```python
from build123d import *

# Parameters (mm, degrees)
F17_DEPTH = 1
F18_DEPTH = 1
F19_DEPTH = 1
F20_DEPTH = 1
F21_DEPTH = 1
F22_DEPTH = 1
F23_DEPTH = 1
F24_DEPTH = 1


with BuildPart() as f17:
    # F4 (on face) → F17 (new body)
    with BuildSketch(Plane(origin=(0, -27.6923076923, 18.4615384615), x_dir=(-1, 0, 0), z_dir=(0, 0.8320502943, -0.5547001962))):
        Polygon((0, -5.0769823397), (0, 49.9230176603), (-5.5, 49.9230176603), (-7, -5.0769823397), align=None)
    extrude(amount=-F17_DEPTH)



with BuildPart() as f18:
    # F6 (on face) → F18 (new body)
    with BuildSketch(Plane(origin=(20.2323563967, -11.4858345379, 8.3203939199), x_dir=(0.4299219493, 0.8853858987, 0.1768019455), z_dir=(0.8188475708, -0.4648567634, 0.3367444808))):
        Polygon((12.9726874522, 53.3990429211), (-21.4851809627, 10.5049255587), (8.4396185165, 12.6277482381), (24.455774925, 43.748203471), align=None)
    extrude(amount=F18_DEPTH)


with BuildPart() as f19:
    # F8 (on face) → F19 (new body)
    with BuildSketch(Plane(origin=(4.8053501819, -15.3618907739, 7.6432203914), x_dir=(-0.9629489756, -0.2414490977, 0.1201316097), z_dir=(-0.2696836488, 0.8621329558, -0.4289492931))):
        Polygon((-14.8009827937, 17.4534178176), (-9.6599579922, 52.0737855798), (-18.5647011331, 53.379752499), (-28.2916584396, 46.352213701), (-42.6343822268, 48.4820668331), (-46.8858296731, 57.5333205922), (-67.1688557163, 60.5080230193), (-62.6933705008, 27.8129158611), align=None)
    extrude(amount=-F19_DEPTH)


with BuildPart() as f20:
    # F10 (on 3pt) → F20 (new body)
    with BuildSketch(Plane(origin=(-9.1548198434, 27.6665002624, 29.3655492724), x_dir=(0.9752092929, 0.1517429862, 0.161061793), z_dir=(-0.2212845115, 0.6687371352, 0.7098054726))):
        Polygon((32.6463562181, -27.0957188494), (23.8535633809, -29.0158214828), (15.0273586911, -41.144222481), (27.5314988539, -50.3037245848), (69.2506974563, -42.194565074), (80.6394600631, -16.615353079), (60.611431934, -20.9889201884), (54.5101233323, -27.6051149669), (43.7738027725, -29.9991535705), align=None)
    extrude(amount=-F20_DEPTH)


with BuildPart() as f21:
    # F12 (on 3pt) → F21 (new body)
    with BuildSketch(Plane(origin=(0, 25.9269177768, 14.9071230511), x_dir=(-1, 0, 0), z_dir=(0, 0.866918652, 0.4984496473))):
        Polygon((-5.5, 52.0151191187), (0, 52.0151191187), (0, 61.5834322338), (-17.6941536866, 61.5834322338), align=None)
    extrude(amount=-F21_DEPTH)


with BuildPart() as f22:
    # F14 (on face) → F22 (new body)
    with BuildSketch(Plane(origin=(0, -4.8915048648, 0.0087522318), x_dir=(1, 0, 0), z_dir=(0, -0.9999983993, 0.001789269))):
        Polygon((0, 85.6087991728), (0, 68.2863061845), (17.6941536866, 68.2863061845), (25.5, 85.6087991728), align=None)
    extrude(amount=F22_DEPTH)


with BuildPart() as f23:
    # F16 (on 3pt) → F23 (new body)
    with BuildSketch(Plane(origin=(0.2488682272, -0.8172223653, -0.1106827247), x_dir=(-0.9573575318, -0.2862919438, -0.0387747249), z_dir=(-0.2889057916, 0.9486959304, 0.1284892032))):
        Polygon((-60.7194634198, 67.8234958605), (-18.2223306139, 68.3171589865), (-26.3758637032, 85.4787410279), (-69.3695216955, 84.7402476712), align=None)
    extrude(amount=-F23_DEPTH)


with BuildPart() as f17_1:
    add(f17.part)

    add(f18.part)  # F24 merges F18

    add(f19.part)  # F24 merges F19

    add(f20.part)  # F24 merges F20

    add(f21.part)  # F24 merges F21

    add(f22.part)  # F24 merges F22

    add(f23.part)  # F24 merges F23
    # F4 (on face) + F6 (on face) + F8 (on face) + F10 (on 3pt) + F12 (on 3pt) + F14 (on face) + F16 (on 3pt) → F24 (join)
    with BuildSketch(Plane(origin=(0, -27.6923076923, 18.4615384615), x_dir=(-1, 0, 0), z_dir=(0, 0.8320502943, -0.5547001962))):
        Polygon((0, -5.0769823397), (0, 49.9230176603), (-5.5, 49.9230176603), (-7, -5.0769823397), align=None)
    with BuildSketch(Plane(origin=(20.2323563967, -11.4858345379, 8.3203939199), x_dir=(0.4299219493, 0.8853858987, 0.1768019455), z_dir=(0.8188475708, -0.4648567634, 0.3367444808))):
        Polygon((12.9726874522, 53.3990429211), (-21.4851809627, 10.5049255587), (8.4396185165, 12.6277482381), (24.455774925, 43.748203471), align=None)
    with BuildSketch(Plane(origin=(4.8053501819, -15.3618907739, 7.6432203914), x_dir=(-0.9629489756, -0.2414490977, 0.1201316097), z_dir=(-0.2696836488, 0.8621329558, -0.4289492931))):
        Polygon((-14.8009827937, 17.4534178176), (-9.6599579922, 52.0737855798), (-18.5647011331, 53.379752499), (-28.2916584396, 46.352213701), (-42.6343822268, 48.4820668331), (-46.8858296731, 57.5333205922), (-67.1688557163, 60.5080230193), (-62.6933705008, 27.8129158611), align=None)
    with BuildSketch(Plane(origin=(-9.1548198434, 27.6665002624, 29.3655492724), x_dir=(0.9752092929, 0.1517429862, 0.161061793), z_dir=(-0.2212845115, 0.6687371352, 0.7098054726))):
        Polygon((32.6463562181, -27.0957188494), (23.8535633809, -29.0158214828), (15.0273586911, -41.144222481), (27.5314988539, -50.3037245848), (69.2506974563, -42.194565074), (80.6394600631, -16.615353079), (60.611431934, -20.9889201884), (54.5101233323, -27.6051149669), (43.7738027725, -29.9991535705), align=None)
    with BuildSketch(Plane(origin=(0, 25.9269177768, 14.9071230511), x_dir=(-1, 0, 0), z_dir=(0, 0.866918652, 0.4984496473))):
        Polygon((-5.5, 52.0151191187), (0, 52.0151191187), (0, 61.5834322338), (-17.6941536866, 61.5834322338), align=None)
    with BuildSketch(Plane(origin=(0, -4.8915048648, 0.0087522318), x_dir=(1, 0, 0), z_dir=(0, -0.9999983993, 0.001789269))):
        Polygon((0, 85.6087991728), (0, 68.2863061845), (17.6941536866, 68.2863061845), (25.5, 85.6087991728), align=None)
    with BuildSketch(Plane(origin=(0.2488682272, -0.8172223653, -0.1106827247), x_dir=(-0.9573575318, -0.2862919438, -0.0387747249), z_dir=(-0.2889057916, 0.9486959304, 0.1284892032))):
        Polygon((-60.7194634198, 67.8234958605), (-18.2223306139, 68.3171589865), (-26.3758637032, 85.4787410279), (-69.3695216955, 84.7402476712), align=None)
    extrude(amount=-F24_DEPTH, dir=(0, 0.8320502943, -0.5547001962))

    # F25: F17 across plane


with BuildPart() as f17_2:
    add(f17_1.part)
    add(f17_1.part.mirror(Plane.YZ))


solid = f17_2.part
```
For this review, take the finished solid that the model builds, in its own axes (mm). A direction names the side the tool comes from. Give positions to 0.01 mm unless a question says otherwise; leave off trailing zeros. Order: outer loops, then holes, each group sorted by start corner. A loop starts at its lowest first (then second) coordinate and runs counter-clockwise, first axis right, second up.
1) Take a section at C-C (x = -3.5). Give the boundary of the cut face in (y, z).
2) The part is to be moulded in two halves that separate along X. For faces 1 (the face through (-6.326, -13.581, 40.947)), 2 (the face through (13.35, -17.68, 17.98)), 3 (the face through (-42.57, 3.76, 23.49)), say which applies: released by +X, released by -X, zero draft, split by the parting line, or undercut.
3) Wall thickness on line 1 (Z direction, x = 56, y = 22); line 2 (X direction, y = 1, z = 49.5); line 3 (X direction, y = -6.5, z = 27): over which ranges is each line inside the solid? List them lowest first.
4) For faces 4 (the face through (-10.279, -10.456, 33.947)), 5 (the face through (-47.878, 18.612, 49.944)), 6 (the face through (-37.226, 9.702, 59.341)), list the 3-axis set-ups (+Z, -Z, +X, -X, +Y, -Y) from which the entire face can be reached by the end or side of a thin tool; tool diameter is ignored.
5) Take a section at B-B (y = 18.5). Give the boundary of the cut face in (x, z), then the cut area to 3 significant figures.
6) Take a section at A-A (x = -39.5). Give the boundary of the cut face in (y, z) (3 decimals).
7) Take a section at D-D (z = 42.5). Give the boundary of the cut face in (x, y).
8) Insertion check: pin 1 (5 mm diameter, centred on x = -7, z = 43.5, fed in from -Y); pin 2 (8 mm diameter, centred on x = 18.5, y = -17.5, fed in from -Z); pin 3 (2 mm diameter, centred on x = -40.5, y = 9, fed in from +Z); pin 4 (1.5 mm diameter, centred on x = -42, z = 79.5, fed in from -Y). Each pin has a flat end and moves straight along its axis. Give the tip position at first contact, or say it passes through.
Derived:
1. outline: (-31.34, 14.79) - (-30.51, 14.24) - (0, 60) - (-4.77, 68.29) - (-4.74, 85.62) - (-5.57, 86.17) - (-5.57, 85.62) - (-5.74, 85.62) - (-5.77, 68.3) - (-5.28, 68.3) - (-5.15, 68.07) - (-5.64, 67.8) - (-1.18, 60.04) - close
2. face 1: undercut
2. face 2: released by +X
2. face 3: released by -X
3. line 1: z = 50.55 to 52.88, 53.61 to 55.02
3. line 2: x = -11.61 to -10.39, 10.39 to 11.61
3. line 3: x = -16.6 to -15.38, 15.38 to 16.6
4. face 4: -Z, +Y
4. face 5: +Y
4. face 6: -X, -Y
5. outline: (-67.43, 38.66) - (-66.92, 36.65) - (-47.46, 48.89) - (-48.13, 50.69) - (-48.38, 50.53) - (-48.42, 50.61) - close; (-64.99, 59.71) - (-47.67, 54.31) - (-46.75, 55.43) - (-64.4, 60.93) - (-64.86, 60.85) - (-64.5, 60.73) - close; (46.75, 55.43) - (47.67, 54.31) - (64.99, 59.71) - (64.5, 60.73) - (64.86, 60.85) - (64.4, 60.93) - close; (47.46, 48.89) - (66.92, 36.65) - (67.43, 38.66) - (48.42, 50.61) - (48.38, 50.53) - (48.13, 50.69) - close
5. area: 140 mm2
6. outline: (-1.554, 85.8) - (0.752, 68.779) - (1.574, 68.888) - (1.667, 68.799) - (1.052, 68.2) - (13.655, 56.326) - (14.395, 57.037) - (1.787, 68.916) - (-0.518, 85.936) - (-1.35, 86.49) - (-1.262, 85.839) - close; (2.201, 23.461) - (3.158, 23.052) - (14.497, 45.843) - (13.665, 46.398) - (13.591, 46.249) - (13.549, 46.268) - close
7. outline: (-68, 20.59) - (-16.45, 4.46) - (-6.9, -12.36) - (-6.55, -12.06) - (-6.09, -12.87) - (6.09, -12.87) - (6.55, -12.06) - (6.9, -12.36) - (16.45, 4.46) - (68, 20.59) - (67.8, 21.69) - (15.77, 5.41) - (6.07, -11.67) - (-6.07, -11.67) - (-15.77, 5.41) - (-67.8, 21.69) - close
8. pin 1: stops at y = -13.77
8. pin 2: passes through
8. pin 3: stops at z = 63.42
8. pin 4: stops at y = -0.19
